from build123d import *

# Parameters (mm, degrees)
BOSS_EXTRUDE1_DEPTH = 2.7
BOSS_EXTRUDE2_START = 2.7
SKETCH1_4_R         = 36.25
BOSS_EXTRUDE2_DEPTH = 2.7


with BuildPart() as part:
    # Sketch1 → Boss-Extrude1 (new body)
    with BuildSketch(Plane.XY):
        with BuildLine():
            Line((-0.00454753, -3.681705965), (151.99545247, -3.681705965))
            ThreePointArc((151.99545247, -3.681705965), (154.823879594, -2.510133089), (155.99545247, 0.318294035))
            Line((155.99545247, 0.318294035), (155.99545247, 191.602313493))
            ThreePointArc((155.99545247, 191.602313493), (154.823879594, 194.430740617), (151.99545247, 195.602313493))
            Line((151.99545247, 195.602313493), (-0.00454753, 195.602313493))
            ThreePointArc((-0.00454753, 195.602313493), (-2.832974655, 194.430740617), (-4.00454753, 191.602313493))
            Line((-4.00454753, 191.602313493), (-4.00454753, 0.318294035))
            ThreePointArc((-4.00454753, 0.318294035), (-2.832974655, -2.510133089), (-0.00454753, -3.681705965))
        make_face()
    extrude(amount=-BOSS_EXTRUDE1_DEPTH)

    # Sketch1_4 → Boss-Extrude2 (add)
    with BuildSketch(Plane.XY.offset(BOSS_EXTRUDE2_START)):
        with BuildLine():
            Line((-4.00454753, 191.602313493), (-4.00454753, 64.175623566))
            Line((-4.00454753, 64.175623566), (-0.00454753, 64.175623566))
            Line((-0.00454753, 64.175623566), (-0.00454753, 187.602313493))
            ThreePointArc((-0.00454753, 187.602313493), (1.167025345, 190.430740617), (3.99545247, 191.602313493))
            Line((3.99545247, 191.602313493), (147.99545247, 191.602313493))
            ThreePointArc((147.99545247, 191.602313493), (150.823879594, 190.430740617), (151.99545247, 187.602313493))
            Line((151.99545247, 187.602313493), (151.99545247, 64.175623566))
            Line((151.99545247, 64.175623566), (155.99545247, 64.175623566))
            Line((155.99545247, 64.175623566), (155.99545247, 191.602313493))
            ThreePointArc((155.99545247, 191.602313493), (154.823879594, 194.430740617), (151.99545247, 195.602313493))
            Line((151.99545247, 195.602313493), (-0.00454753, 195.602313493))
            ThreePointArc((-0.00454753, 195.602313493), (-2.832974655, 194.430740617), (-4.00454753, 191.602313493))
        make_face()
        with Locations(Location((75.99545247, 95.960303764, 0), (0, 0, 180))):
            Circle(SKETCH1_4_R)
    extrude(amount=-BOSS_EXTRUDE2_DEPTH)


solid = part.part
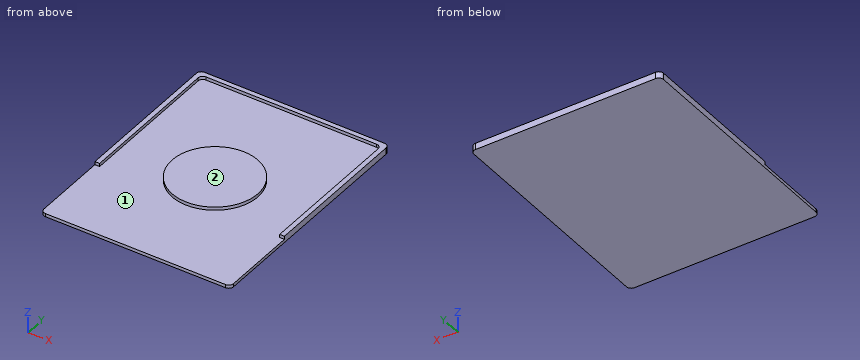
Verification items for the finished model (mm, model axes). Face numbers are marked on the shaded views. Give positions to 0.01 mm unless a question says otherwise; leave off trailing zeros. Write each loop counter-clockwise with the first axis right and the second up, starting at its lowest first coordinate (ties: lowest second). Pieces come first, ordered by that corner, then holes. Notation, with made-up numbers: M 31.25,17.25 L 39.25,17.25 A26 ccw 39.25,37.25 Z; hole C 56,-23 d11. An arc over 180 degrees is marked long. Put each result on its own line as item: value. Start each with the question number.
1. Section check A-A (y = 168.5). Record the cut outline in (x, z), and give its area (3 significant figures).
2. Section check B-B (x = 25.5). Record the cut outline in (y, z).
3. Section check C-C (z = 1.65). Record the cut outline in (x, y), and give its area (3 significant figures).
4. Section check D-D (x = 54). Record the cut outline in (y, z).
5. Go/stop test with flat-tipped pins: pin 1 Ø5 at (x, y) = (67.5, 39) entering from +Z; pin 2 Ø1.4 at (x, z) = (-2.5, 1) entering from -Y; pin 3 Ø3 at (x, z) = (100, 2) entering from -Y. Record where each tip stops, or that it passes through.
6. Draft check along Y on the marked faces 1 and 2. Enter one of: +Y half, -Y half, draft (parallel to the pull), parting line (faces both ways), or undercut.
7. Scan lines: line 1 along X through (y, z) = (146, 1.8); line 2 along X through (y, z) = (113, 1); line 3 along X through (y, z) = (93, 2.4). Record each from-to range of solid material in increasing order. Write a range as [from, to].
Answer list:
1. outline: M -4,-2.7 L 156,-2.7 L 156,2.7 L 152,2.7 L 152,0 L 0,0 L 0,2.7 L -4,2.7 Z
1. area: 454 mm2
2. outline: M -3.68,-2.7 L 195.6,-2.7 L 195.6,2.7 L 191.6,2.7 L 191.6,0 L -3.68,0 Z
3. outline: M -4,64.18 L 0,64.18 L 0,187.6 A4 cw 4,191.6 L 148,191.6 A4 cw 152,187.6 L 152,64.18 L 156,64.18 L 156,191.6 A4 ccw 152,195.6 L 0,195.6 A4 ccw -4,191.6 Z; C 76,95.96 d72.5
3. area: 5,790 mm2
4. outline: M -3.68,-2.7 L 195.6,-2.7 L 195.6,2.7 L 191.6,2.7 L 191.6,0 L 124.77,0 L 124.77,2.7 L 67.15,2.7 L 67.15,0 L -3.68,0 Z
5. pin 1: z = 0
5. pin 2: y = 64.18
5. pin 3: y = 67.54
6. face 1: undercut
6. face 2: draft
7. line 1: [-4, 0], [152, 156]
7. line 2: [-4, 0], [44, 107.99], [152, 156]
7. line 3: [-4, 0], [39.87, 112.12], [152, 156]
